Design review of the part shown in the three views and the two pictorial views. Dimensions are in mm from the part's minimum x, y and z. A direction names the side the tool comes from. Give positions to 0.01 mm unless a question says otherwise; leave off trailing zeros. Order: outer loops, then holes, each group sorted by start corner. A loop starts at its lowest first (then second) coordinate and runs counter-clockwise, first axis right, second up. Notation, with made-up numbers: M -33.75,22 L 21.25,22 A15 ccw 21.25,26 Z; hole C -9,2 d5. An arc over 180 degrees is marked long. Answer as a JSON object with one key per item and string values.
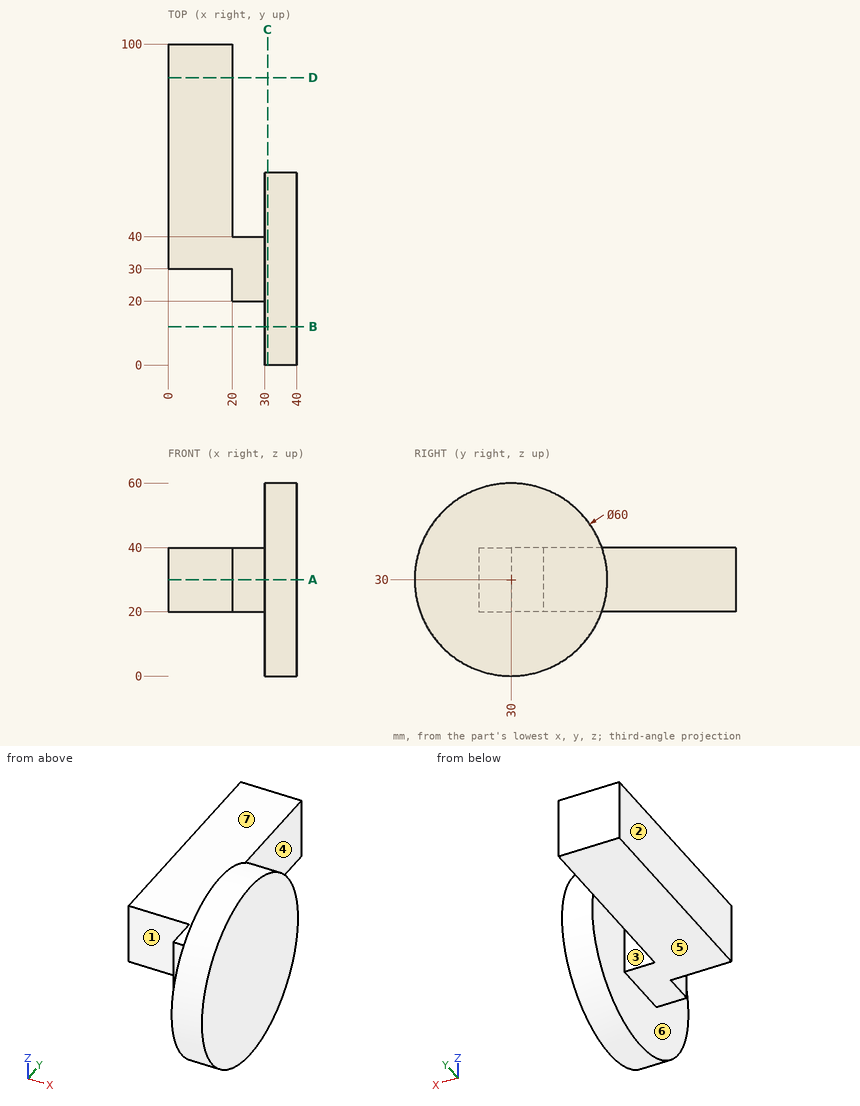
(1) We need section A-A (z = 30). Write out the cut boundary in (x, y).
Checked values:
{"outline": "M 0,30 L 20,30 L 20,20 L 30,20 L 30,0 L 40,0 L 40,60 L 30,60 L 30,40 L 20,40 L 20,100 L 0,100 Z"}
(2) Insertion check: pin 1 (11 mm diameter, centred on y = 23.5, z = 27, fed in from -X); pin 2 (8 mm diameter, centred on x = 21.5, y = 27, fed in from -Z); pin 3 (11 mm diameter, centred on x = 24, z = 31.5, fed in from -Y). Each pin has a flat end and moves straight along its axis. Give the tip position at first contact, or say it passes through.
Checked values:
{"pin 1": "stops at x = 20", "pin 2": "stops at z = 20", "pin 3": "stops at y = 20"}
(3) We need section D-D (y = 89.5). Write out the cut boundary in (x, z).
Checked values:
{"outline": "M 0,20 L 20,20 L 20,40 L 0,40 Z"}
(4) We need section B-B (y = 12). Write out the cut boundary in (x, z), plus the area to 3 significant figures.
Checked values:
{"outline": "M 30,6 L 40,6 L 40,54 L 30,54 Z", "area": "480 mm^2"}
(5) Tool access review of the marked faces 5, 6 and 7: name each direction out of +Z, -Z, +X, -X, +Y, -Y from which nothing blocks a thin tool from reaching the whole face with its end or side.
Checked values:
{"face 5": "-Z, -X, +Y, -Y", "face 6": "none", "face 7": "+Z, -X, +Y, -Y"}
(6) To check wall thickness, follow L1, parallel to X at y = 36.5, z = 46.5; L2, parallel to Z at x = 19, y = 70.5; L3, parallel to Y at x = 12, z = 24. State the ranges of each line that lie inside material, in increasing order. Write a range as from..to.
Checked values:
{"L1": "x = 30..40", "L2": "z = 20..40", "L3": "y = 30..100"}
(7) Draft analysis for pull direction X (two halves, no side actions). For the marked faces 1, 2, 3 and 4, state which applies: +X half, -X half, draft (parallel to the pull), parting line (faces both ways), or undercut.
Checked values:
{"face 1": "draft", "face 2": "-X half", "face 3": "undercut", "face 4": "undercut"}
(8) We need section C-C (x = 31). Write out the cut boundary in (y, z).
Checked values:
{"outline": "C 30,30 d60"}
